Input: part model. Units: mm. Frame: model coordinates. A direction names the side the tool comes from. Give positions to 0.01 mm unless a question says otherwise; leave off trailing zeros. Loops run counter-clockwise (first coordinate to the right, second up) from the corner with the lowest first, then second, coordinate; pieces in that order, holes last. Notation, with made-up numbers: (-10.75, 50.25) -> (45.25, 50.25) arc R21 cw to (45.25, 64.25) -> close; hole circle Ø8 at (63.5, 61). An arc over 180 degrees is marked (long way). Answer as a JSON object with one key per item and string values.
```python
from build123d import *

# Parameters (mm, degrees)
SKETCH1_R               = 25
BOSS_EXTRUDE1_DEPTH     = 10
SKETCH2_R               = 20
CUT_EXTRUDE1_DEPTH      = 2
SKETCH3_R               = 6.625
CUT_EXTRUDE2_DEPTH      = 5
SKETCH4_R               = 3.75
CUT_EXTRUDE4_DEPTH      = 8
CUT_EXTRUDE4_DEPTH_BACK = 4


with BuildPart() as part:
    # Sketch1 → Boss-Extrude1 (new body)
    with BuildSketch(Plane(origin=(0, 0, 0), x_dir=(1, 0, 0), z_dir=(0, 1, 0))):
        Circle(SKETCH1_R)
    extrude(amount=BOSS_EXTRUDE1_DEPTH)

    # Sketch2 → Cut-Extrude1 (cut)
    with BuildSketch(Plane(origin=(0, 10, 0), x_dir=(1, 0, 0), z_dir=(0, 1, 0))):
        Circle(SKETCH2_R)
    extrude(amount=-CUT_EXTRUDE1_DEPTH, mode=Mode.SUBTRACT)

    # Sketch3 → Cut-Extrude2 (cut)
    with BuildSketch(Plane(origin=(0, 8, 0), x_dir=(1, 0, 0), z_dir=(0, 1, 0))):
        Circle(SKETCH3_R)
    extrude(amount=-CUT_EXTRUDE2_DEPTH, mode=Mode.SUBTRACT)

    # Sketch4 → Cut-Extrude4 (cut, two sides)
    with BuildSketch(Plane(origin=(0, 3, 0), x_dir=(1, 0, 0), z_dir=(0, 1, 0))) as cut_extrude4_sk:
        Circle(SKETCH4_R)
    extrude(amount=CUT_EXTRUDE4_DEPTH, mode=Mode.SUBTRACT)
    extrude(cut_extrude4_sk.sketch, amount=-CUT_EXTRUDE4_DEPTH_BACK, mode=Mode.SUBTRACT)


solid = part.part
```
Q1. Section A-A, the plane z = 0. Return the cut outline in (x, y) (3 decimals).
Evaluation:
{"outline": "(-25, 0) -> (-3.75, 0) -> (-3.75, 3) -> (-6.625, 3) -> (-6.625, 8) -> (-20, 8) -> (-20, 10) -> (-25, 10) -> close; (3.75, 0) -> (25, 0) -> (25, 10) -> (20, 10) -> (20, 8) -> (6.625, 8) -> (6.625, 3) -> (3.75, 3) -> close"}
Q2. Ray query, line 1 along X through (y, z) = (1.1, 0); line 2 along Z through (x, y) = (0, 9.55); line 3 along X through (y, z) = (4.2, 0) (3 decimals). Return the intervals inside material, ascending.
Evaluation:
{"line 1": "x = -25 to -3.75, 3.75 to 25", "line 2": "z = -25 to -20, 20 to 25", "line 3": "x = -25 to -6.625, 6.625 to 25"}
Q3. Section B-B, the plane x = 0. Return the cut outline in (y, z) (3 decimals).
Evaluation:
{"outline": "(0, -25) -> (10, -25) -> (10, -20) -> (8, -20) -> (8, -6.625) -> (3, -6.625) -> (3, -3.75) -> (0, -3.75) -> close; (0, 3.75) -> (3, 3.75) -> (3, 6.625) -> (8, 6.625) -> (8, 20) -> (10, 20) -> (10, 25) -> (0, 25) -> close"}
Q4. Pin query (flat end, axial travel): pin 1 (7 mm diameter, centred on x = 0, z = 0, fed in from +Y); pin 2 (21 mm diameter, centred on x = 0, z = 0, fed in from +Y); pin 3 (6 mm diameter, centred on y = 7.5, z = 5.5, fed in from +X); pin 4 (2 mm diameter, centred on y = 2.5, z = -1.5, fed in from -X) (3 decimals). Return the tip coordinate at first contact, or that it passes through.
Evaluation:
{"pin 1": "passes through", "pin 2": "stops at y = 8", "pin 3": "stops at x = 24.87", "pin 4": "stops at x = -24.995"}
Q5. Access query for faces 5 (the cylindrical face through (3.562, 5.535, -5.586)), 6 (the flat face through (-11, 10, -17)). Directions: +Z, -Z, +X, -X, +Y, -Y. A direction counts if a zero-diameter tool reaches every point of the face in a straight line with its end or side. Return the directions, or none.
Evaluation:
{"face 5": "+Y", "face 6": "+Z, -Z, +X, -X, +Y"}
Q6. Draft query along Z for faces 1 (the cylindrical face through (-3.746, 1.521, -0.165)), 2 (the flat face through (0, 0, 5)), 3 (the cylindrical face through (23.846, 4.93, -7.509)), 4 (the cylindrical face through (-4.336, 9.014, 19.524)). Return one class per face: +Z half, -Z half, draft (parallel to the pull), parting line (faces both ways), or undercut.
Evaluation:
{"face 1": "undercut", "face 2": "draft", "face 3": "parting line", "face 4": "undercut"}
Q7. Section D-D, the plane x = 17.5. Return the cut outline in (y, z), then the cut area to 3 significant figures.
Evaluation:
{"outline": "(0, -17.85) -> (10, -17.85) -> (10, -9.68) -> (8, -9.68) -> (8, 9.68) -> (10, 9.68) -> (10, 17.85) -> (0, 17.85) -> close", "area": "318 mm2"}
Q8. Section C-C, the plane y = 4.5. Return the cut outline in (x, z) (3 decimals), then the cut area to 3 significant figures.
Evaluation:
{"outline": "circle Ø50 at (0, 0); hole circle Ø13.25 at (0, 0)", "area": "1,830 mm2"}
